from build123d import *

# Parameters (mm, degrees)
SKETCH1_W           = 40
SKETCH1_H           = 30
BOSS_EXTRUDE2_DEPTH = 60
SKETCH3_W           = 10
SKETCH3_H           = 30
CUT_EXTRUDE1_DEPTH  = 60
CUT_EXTRUDE2_DEPTH  = 60
CUT_EXTRUDE3_DEPTH  = 60
CUT_EXTRUDE4_DEPTH  = 60
BOSS_EXTRUDE7_DEPTH = 0.0001


with BuildPart() as part:
    # Sketch1 → Boss-Extrude2 (new body)
    with BuildSketch(Plane.XY):
        Polygon((50, 30), (20, 60), (-10, 30), (0, 30), (40, 30), align=None)
        with Locations((20, 15)):
            Rectangle(SKETCH1_W, SKETCH1_H)
    extrude(amount=BOSS_EXTRUDE2_DEPTH)

    # Sketch3 → Cut-Extrude1 (cut)
    with BuildSketch(Plane(origin=(0, 0, 0), x_dir=(0, 0, -1), z_dir=(1, 0, 0))):
        Polygon((-30, 60), (0, 60), (0, 30), align=None)
        Polygon((-60, 30), (-60, 60), (-30, 60), align=None)
        with Locations((-5, 15)):
            Rectangle(SKETCH3_W, SKETCH3_H)
        with Locations((-55, 15)):
            Rectangle(SKETCH3_W, SKETCH3_H)
    extrude(amount=CUT_EXTRUDE1_DEPTH, mode=Mode.SUBTRACT)

    # Sketch4 → Cut-Extrude2 (cut)
    with BuildSketch(Plane(origin=(0, 0, 0), x_dir=(0, 0, -1), z_dir=(1, 0, 0))):
        Polygon((-60, 30), (-50, 40), (-60, 40), align=None)
    extrude(amount=-CUT_EXTRUDE2_DEPTH, mode=Mode.SUBTRACT)

    # Sketch5 → Cut-Extrude3 (cut)
    with BuildSketch(Plane(origin=(0, 0, 0), x_dir=(0, 0, -1), z_dir=(1, 0, 0))):
        Polygon((-10, 40), (0, 40), (0, 30), align=None)
    extrude(amount=-CUT_EXTRUDE3_DEPTH, mode=Mode.SUBTRACT)

    # Sketch6 → Cut-Extrude4 (cut)
    with BuildSketch(Plane(origin=(0, 60, 0), x_dir=(1, 0, 0), z_dir=(0, 1, 0))):
        Polygon((-10, 0), (-10, -60), (50, -60), align=None)
    extrude(amount=-CUT_EXTRUDE4_DEPTH, mode=Mode.SUBTRACT)

    # Sketch7 → Boss-Extrude7 (add)
    with BuildSketch(Plane.XZ):
        with BuildLine():
            Line((0, 10), (40, 10))
            Line((40, 10), (40, 50))
            ThreePointArc((40, 50), (11.715728753, 38.284271247), (0, 10))
        make_face()
    extrude(amount=-BOSS_EXTRUDE7_DEPTH)


solid = part.part
Build history of the part. All positions in model axes, mm. A direction names the side the tool comes from. Round coordinates to 2 decimals unless told otherwise and drop trailing zeros. Write each loop counter-clockwise with the first axis right and the second up, starting at its lowest first coordinate (ties: lowest second). Pieces come first, ordered by that corner, then holes. Notation, with made-up numbers: M 11.5,66.25 L 40.5,66.25 A27 ccw 40.5,93.25 Z; hole C -5,66 d2. An arc over 180 degrees is marked long. Answer as a JSON object with one key per item and string values. Group by question number.
(1) Which spindle directions (+Z, -Z, +X, -X, +Y, -Y) get a long thin tool onto all of the face, cutting with end or side? Do faces 1 (the flat face through (20, 15, 10)), 2 (the flat face through (20, 41, 11)), 3 (the flat face through (40, 15, 30)), 4 (the flat face through (20, 24, 30)), 5 (the flat face through (24, 0, 25)). Say none if no direction does.
(2) Drill centre lines: L1, parallel to Z at x = 14, y = 48.5; L2, parallel to Y at x = 44, z = 14; L3, parallel to X at y = 34, z = 15.5. Where is each one in solid material? Low to high.
(3) Cut at C-C (y = 41). Give the cut face in (x, z), and give its area (3 significant figures).
(4) Flat gauge pins, fed straight in: pin 1 (2 mm diameter, centred on y = 45, z = 36, fed in from -X); pin 2 (9 mm diameter, centred on y = 21, z = 28.5, fed in from +X); pin 3 (9 mm diameter, centred on x = 26, y = 14, fed in from -Z). Where does each tip first touch, or does it go through?
Responses:
{
 "1": {"face 1": "-Z, +X, -X, -Y", "face 2": "-Z, +X, -X, +Y", "face 3": "+Z, -Z, +X, -Y", "face 4": "+Z, -X, +Y", "face 5": "+Z, -Z, +X, -X, -Y"},
 "2": {"L1": "z = 18.5 to 24", "L2": "y = 30 to 36", "L3": "x = 5.5 to 46"},
 "3": {"outline": "M 1,11 L 39,11 L 39,49 Z", "area": "722 mm2"},
 "4": {"pin 1": "stops at x = 25", "pin 2": "stops at x = 40", "pin 3": "stops at z = 10"}
}
